Autodesk Inventor part; units mm, degrees
ref_plane "YZ Plane" through (0, 0, 0) normal (1, 0, 0) x (0, 1, 0)
ref_plane "XZ Plane" through (0, 0, 0) normal (0, 1, 0) x (-1, 0, 0)
ref_plane "XY Plane" through (0, 0, 0) normal (0, 0, 1) x (1, 0, 0)
sketch "スケッチ1" plane through (0, 0, 0) normal (0, 0, 1) x (1, 0, 0)
  line L0 (17.8, -27.8) -> (17.8, 27.8)
  arc A0 (17.8, 27.8) -> (14.8, 30.8) centre (14.8, 27.8) ccw
  line L1 (14.8, 30.8) -> (-14.8, 30.8)
  arc A1 (-14.8, 30.8) -> (-17.8, 27.8) centre (-14.8, 27.8) ccw
  line L2 (-17.8, 27.8) -> (-17.8, -27.8)
  arc A2 (-17.8, -27.8) -> (-14.8, -30.8) centre (-14.8, -27.8) ccw
  line L3 (-14.8, -30.8) -> (14.8, -30.8)
  arc A3 (14.8, -30.8) -> (17.8, -27.8) centre (14.8, -27.8) ccw
  point P0 (0, 0)
extrude "押し出し1" add sketch "スケッチ1" along normal blind 15
fillet "フィレット1" radius 3 8 edges at (-16.9213, 29.9213, 15) (-17.8, 0, 15) (-16.9213, -29.9213, 15) (0, -30.8, 15) (16.9213, -29.9213, 15) (17.8, 0, 15) (16.9213, 29.9213, 15) (0, 30.8, 15)
shell "シェル1" thickness 0.8 removed faces 1 at (5.9333, 9.2667, 0)
sketch "スケッチ2" plane through (17.8, -27.8, 0) normal (1, 0, 0) x (0, 0, -1)
  line L0 (0, 51.6) -> (-6, 51.6)
  line L1 (-6, 51.6) -> (-6, 38.6)
  line L2 (-6, 38.6) -> (0, 38.6)
  line L3 (0, 38.6) -> (0, 51.6)
  line L4 (0, 58.6) -> (-12, 58.6)
  line L5 (0, 0) -> (0, 55.6)
  point P0 (0, 27.8)
  dimension "d4" = 6
  dimension "d5" = 7
  dimension "d6" = 20
extrude "押し出し2" cut sketch "スケッチ2" against normal blind 15
fillet "フィレット2" radius 1.5 2 edges at (17.4, 10.8, 6) (17.4, 23.8, 6)
sketch "スケッチ3" plane through (0, 0, 15) normal (0, 0, 1) x (1, 0, 0)
  line L0 (-17.8, 27.8) -> (-17.8, -27.8)
  line L1 (-14.8, -30.8) -> (14.8, -30.8)
  line L2 (17.8, -27.8) -> (17.8, 27.8)
  line L3 (14.8, 30.8) -> (-14.8, 30.8)
  circle A0 centre (-3.8, 11.8) radius 6.15
  circle A1 centre (-3.8, -16.8) radius 2.65
  circle A2 centre (-3.8, -4.2) radius 6.65
  circle A3 centre (-3.8, -23.8) radius 1.15
  point P0 (0, 0)
  dimension "d10" = 12.3
  dimension "d11" = 19
  dimension "d12" = 14
  dimension "d14" = 5.3
  dimension "d15" = 13.3
  dimension "d16" = 2.3
  dimension "d17" = 14
  dimension "d18" = 14
  dimension "d19" = 7
  dimension "d20" = 14
  dimension "d21" = 14
  dimension "d22" = 35
extrude "押し出し3" cut sketch "スケッチ3" against normal blind 15
fillet "フィレット3" radius 1 4 edges at (-4.95, -23.8, 15) (-6.45, -16.8, 15) (-10.45, -4.2, 15) (-9.95, 11.8, 15)
Could you check a few things on this model? Use its own coordinates, in mm. A direction names the side the tool comes from. Give positions to 0.01 mm unless a question says otherwise; leave off trailing zeros. Order: outer loops, then holes, each group sorted by start corner. A loop starts at its lowest first (then second) coordinate and runs counter-clockwise, first axis right, second up.
Q1. I'm going to push flat-ended pins straight in: P1, Ø1, axis at x = -1, y = 24.5, coming from the -Z side; P2, Ø6, axis at x = -13.5, y = -23.5, coming from the -Z side; P3, Ø0.9, axis at x = 17.5, z = 2, coming from the +Y side. Where does each tip first touch, or does it pass through?
Q2. Suppose I cut it at A-A, the plane z = 11. Write out the boundary of the cut face in (x, y).
Q3. Suppose I cut it at D-D, the plane z = 2. Write out the boundary of the cut face in (x, y), and give its area (3 significant figures).
Q4. We'd pull the mould along Y, two halves only. Please class faces 3 (the flat face through (-17, 0, 6)), 4 (the flat face through (-17.2, -2.1, 0)), 5 (the cylindrical face through (-16.94, 29.9, 5.92)): +Y half, -Y half, draft (parallel to the pull), parting line (faces both ways), or undercut.
Q5. If I drill on line 1 along Y through (x, z) = (-5, 9.5); line 2 along X through (y, z) = (-26, 3.5); line 3 along Z through (x, y) = (-11, -24), over which ranges is the centre line in solid material (lowest first)?
Q6. For faces 1 (the flat face through (-17.8, 0, 6)), 2 (the flat face through (17, 0, 6)), which set-ups out of +Z, -Z, +X, -X, +Y, -Y let a thin tool reach every point of the face, with its end or its side?
Q7. Suppose I cut it at B-B, the plane y = 21.5. Write out the boundary of the cut face in (x, z), and give its area (3 significant figures).
Q8. Suppose I cut it at C-C, the plane x = 5.5. Write out the boundary of the cut face in (y, z), and give its area (3 significant figures).
Solution:
1. P1: stops at z = 14.2
1. P2: stops at z = 13.4
1. P3: stops at y = 29.78
2. outline: (-17.8, -27.8) arc R3 ccw to (-14.8, -30.8) - (14.8, -30.8) arc R3 ccw to (17.8, -27.8) - (17.8, 27.8) arc R3 ccw to (14.8, 30.8) - (-14.8, 30.8) arc R3 ccw to (-17.8, 27.8) - close; hole (-17, -27.8) arc R2.2 ccw to (-14.8, -30) - (14.8, -30) arc R2.2 ccw to (17, -27.8) - (17, 27.8) arc R2.2 ccw to (14.8, 30) - (-14.8, 30) arc R2.2 ccw to (-17, 27.8) - close
3. outline: (-17.8, -27.8) arc R3 ccw to (-14.8, -30.8) - (14.8, -30.8) arc R3 ccw to (17.8, -27.8) - (17.8, 10.8) - (17, 10.8) - (17, -27.8) arc R2.2 cw to (14.8, -30) - (-14.8, -30) arc R2.2 cw to (-17, -27.8) - (-17, 27.8) arc R2.2 cw to (-14.8, 30) - (14.8, 30) arc R2.2 cw to (17, 27.8) - (17, 23.8) - (17.8, 23.8) - (17.8, 27.8) arc R3 ccw to (14.8, 30.8) - (-14.8, 30.8) arc R3 ccw to (-17.8, 27.8) - close
3. area: 139 mm2
4. face 3: undercut
4. face 4: draft
4. face 5: +Y half
5. line 1: y = -30.8 to -30, 30 to 30.8
5. line 2: x = -17.8 to -17, 17 to 17.8
5. line 3: z = 14.2 to 15
6. face 1: +Z, -Z, -X, +Y, -Y
6. face 2: -Z
7. outline: (-17.8, 0) - (-17, 0) - (-17, 12) arc R2.2 cw to (-14.8, 14.2) - (14.8, 14.2) arc R2.2 cw to (17, 12) - (17, 6) - (17.8, 6) - (17.8, 12) arc R3 ccw to (14.8, 15) - (-14.8, 15) arc R3 ccw to (-17.8, 12) - close
7. area: 44.6 mm2
8. outline: (-30.8, 0) - (-30, 0) - (-30, 12) arc R2.2 cw to (-27.8, 14.2) - (27.8, 14.2) arc R2.2 cw to (30, 12) - (30, 0) - (30.8, 0) - (30.8, 12) arc R3 ccw to (27.8, 15) - (-27.8, 15) arc R3 ccw to (-30.8, 12) - close
8. area: 70.2 mm2
